```python
from build123d import *

# Parameters (mm, degrees)
EXTRUDE_1_DEPTH          = 6.7
CUT_EXTRUDE_1_DEPTH      = 29.713280899
CUT_EXTRUDE_1_DEPTH_BACK = 29.713280899
SKETCH_2_W               = 5
SKETCH_2_H               = 9
FILLET_1_R               = 1
SKETCH_3_R               = 1.6
CUT_EXTRUDE_2_DEPTH      = 13.4
CUT_EXTRUDE_3_DEPTH      = 31.969702937


with BuildPart() as part:
    # 草图1 → 凸台-拉伸1 (new, symmetric)
    with BuildSketch(Plane(origin=(0, 0, 0), x_dir=(0, 0, -1), z_dir=(1, 0, 0))):
        Polygon((3.15, 0), (-3.15, 0), (-3.15, 8.9), (-9.65, 8.9), (-9.65, 11.7), (-3.15, 11.7), (-3.15, 26.2), (3.15, 26.2), align=None)
    extrude(amount=EXTRUDE_1_DEPTH, both=True)

    # 草图2 → 切除-拉伸1 (cut, two sides: drawn at the far end of the back side and taken through both)
    with BuildSketch(Plane.XY.offset(-CUT_EXTRUDE_1_DEPTH_BACK)):
        with Locations((0, 21.7)):
            Rectangle(SKETCH_2_W, SKETCH_2_H)
    extrude(amount=CUT_EXTRUDE_1_DEPTH + CUT_EXTRUDE_1_DEPTH_BACK, mode=Mode.SUBTRACT)

    # 圆角1
    fillet_1_edges = [part.edges().sort_by_distance(p)[0] for p in [
        (6.7, 10.3, 9.65),
        (-6.7, 10.3, 9.65),
    ]]
    fillet(fillet_1_edges, radius=FILLET_1_R)

    # 草图3 → 切除-拉伸2 (cut)
    with BuildSketch(Plane(origin=(0, 11.7, 0), x_dir=(1, 0, 0), z_dir=(0, 1, 0))):
        with Locations(Location((3.5, -6.65, 0), (0, 0, 270))):
            Circle(SKETCH_3_R)
        with Locations(Location((-3.5, -6.65, 0), (0, 0, 270))):
            Circle(SKETCH_3_R)
    extrude(amount=-CUT_EXTRUDE_2_DEPTH, mode=Mode.SUBTRACT)

    # 草图4 → 切除-拉伸3 (cut, through all)
    with BuildSketch(Plane(origin=(6.7, 0, 0), x_dir=(0, 0, -1), z_dir=(1, 0, 0))):
        with BuildLine():
            Line((0.4, 24.3), (0.4, 22.3))
            ThreePointArc((0.4, 22.3), (0, 21.9), (-0.4, 22.3))
            Line((-0.4, 22.3), (-0.4, 24.3))
            ThreePointArc((-0.4, 24.3), (0, 24.7), (0.4, 24.3))
        make_face()
    extrude(amount=-CUT_EXTRUDE_3_DEPTH, mode=Mode.SUBTRACT)


solid = part.part
```
Can you work these out from the model? Positions are in its coordinate system, mm. A direction names the side the tool comes from. Coordinates: 2 decimals unless noted, no trailing zeros. Loops run counter-clockwise (first coordinate to the right, second up) from the corner with the lowest first, then second, coordinate; pieces in that order, holes last.
Item 1: Suppose I cut it at D-D (y = 10.25). Please give me the cut outline in (x, z), then the cut area to 3 significant figures.
Answers below:
outline: (-6.7, -3.15) - (6.7, -3.15) - (6.7, 8.65) arc R1 ccw to (5.7, 9.65) - (-5.7, 9.65) arc R1 ccw to (-6.7, 8.65) - close; hole circle Ø3.2 at (-3.5, 6.65); hole circle Ø3.2 at (3.5, 6.65)
area: 155 mm2
Item 2: If we mould it in two halves opening along X, with no side actions, what happens to faces 4 (the face through (0, 17.2, 0)), 5 (the face through (6.7, 13, 0)), 6 (the face through (4.6, 21.9, 0)), 7 (the face through (-6.415, 10.32, 9.349))? For each: released by +X, released by -X, zero draft, split by the parting line, or undercut.
Answers below:
face 4: undercut
face 5: released by +X
face 6: zero draft
face 7: released by -X
Item 3: Which directions (+Z, -Z, +X, -X, +Y, -Y) give clear straight access to the entire face, cutting with the end or side of a thin tool? Please do faces 1 (the face through (-5, 23, 0.4)), 2 (the face through (0, 16, 3.15)), 3 (the face through (0, 8.9, 6)).
Answers below:
face 1: +X, -X
face 2: +Z, +X, -X, +Y
face 3: +Z, +X, -X, -Y
Item 4: I'm going to push flat-ended pins straight in: pin 1 (1.6 mm diameter, centred on x = -4.5, y = 23.5, fed in from +Z); pin 2 (3.5 mm diameter, centred on x = -3.5, z = 6.65, fed in from +Y); pin 3 (2 mm diameter, centred on x = 3.5, z = -2, fed in from -Y); pin 4 (4.5 mm diameter, centred on x = 0.5, y = 6.5, fed in from +Z). Where does each tip first touch, or does it pass through?
Answers below:
pin 1: stops at z = 3.15
pin 2: stops at y = 11.7
pin 3: stops at y = 0
pin 4: stops at z = 3.15
Item 5: Suppose I cut it at C-C (x = 1.5). Please give me the cut outline in (y, z).
Answers below:
outline: (0, -3.15) - (17.2, -3.15) - (17.2, 3.15) - (11.7, 3.15) - (11.7, 9.65) - (8.9, 9.65) - (8.9, 3.15) - (0, 3.15) - close
Item 6: Suppose I cut it at A-A (x = 3.5). Please give me the cut outline in (y, z), then the cut area to 3 significant figures.
Answers below:
outline: (0, -3.15) - (26.2, -3.15) - (26.2, 3.15) - (11.7, 3.15) - (11.7, 5.05) - (8.9, 5.05) - (8.9, 3.15) - (0, 3.15) - close; (8.9, 8.25) - (11.7, 8.25) - (11.7, 9.65) - (8.9, 9.65) - close; hole (22.3, -0.4) - (24.3, -0.4) arc R0.4 ccw to (24.3, 0.4) - (22.3, 0.4) arc R0.4 ccw to start
area: 172 mm2
Item 7: Please list where these lines run through material, in increasing order: L1, parallel to X at y = 10, z = 6.65; L2, parallel to X at y = 19.25, z = 0.25; L3, parallel to Y at x = 1.25, z = 6.75.
Answers below:
L1: x = -6.7 to -5.1, -1.9 to 1.9, 5.1 to 6.7
L2: x = -6.7 to -2.5, 2.5 to 6.7
L3: y = 8.9 to 11.7
Item 8: Suppose I cut it at B-B (z = 6.65). Please give me the cut outline in (x, y), then the cut area to 3 significant figures.
Answers below:
outline: (-6.7, 8.9) - (-5.1, 8.9) - (-5.1, 11.7) - (-6.7, 11.7) - close; (-1.9, 8.9) - (1.9, 8.9) - (1.9, 11.7) - (-1.9, 11.7) - close; (5.1, 8.9) - (6.7, 8.9) - (6.7, 11.7) - (5.1, 11.7) - close
area: 19.6 mm2
